```python
from build123d import *

# Parameters (mm, degrees)
F0_R     = 8.9
F3_DEPTH = 13.5
F0_W     = 27.7
F0_H     = 11
F0_H_2   = 1.2
F4_DEPTH = 10.5
F2_R     = 10.7
F5_DEPTH = 5
F2_R_2   = 3.25
F6_DEPTH = 2
F2_R_3   = 3
F7_DEPTH = 6
F8_DEPTH = 5.5
F9_SIZE  = 1
F10_SIZE = 2
F11_R    = 0.2


with BuildPart() as f3:
    # F0 (on Top) → F3 (new body)
    with BuildSketch(Plane.XY):
        with BuildLine():
            Line((0, 19.0066603875), (0, 0))
            Line((0, 0), (18.3, 0))
            Line((18.3, 0), (18.3, 18.5502631652))
            ThreePointArc((18.3, 18.5502631652), (17.5, 23.3), (18.3, 28.0497368348))
            Line((18.3, 28.0497368348), (18.3, 36.8))
            Line((18.3, 36.8), (0, 36.8))
            Line((0, 36.8), (0, 27.5933396125))
            Line((0, 27.5933396125), (3.4058666579, 26.680740392))
            ThreePointArc((3.4058666579, 26.680740392), (6, 23.3), (3.4058666579, 19.919259608))
            Line((3.4058666579, 19.919259608), (0, 19.0066603875))
        make_face()
        with BuildLine():
            Line((18.3, 18.5502631652), (18.3, 0))
            Line((18.3, 0), (35.3, 0))
            Line((35.3, 0), (35.3, 7))
            ThreePointArc((35.3, 7), (36.4715728753, 9.8284271247), (39.3, 11))
            Line((39.3, 11), (64.3, 11))
            Line((64.3, 11), (64.3, 35.6))
            Line((64.3, 35.6), (39.3, 35.6))
            ThreePointArc((39.3, 35.6), (37.7508066615, 35.9121822171), (36.4434286286, 36.8))
            Line((36.4434286286, 36.8), (18.3, 36.8))
            Line((18.3, 36.8), (18.3, 28.0497368348))
            ThreePointArc((18.3, 28.0497368348), (17.5, 23.3), (18.3, 18.5502631652))
        make_face()
        with Locations((32, 23.3)):
            Circle(F0_R, mode=Mode.SUBTRACT)
        with BuildLine():
            Line((64.3, 35.6), (64.3, 11))
            Line((64.3, 11), (92, 11))
            Line((92, 11), (92, 19.0066603875))
            Line((92, 19.0066603875), (88.5941333421, 19.919259608))
            ThreePointArc((88.5941333421, 19.919259608), (86, 23.3), (88.5941333421, 26.680740392))
            Line((88.5941333421, 26.680740392), (92, 27.5933396125))
            Line((92, 27.5933396125), (92, 35.6))
            Line((92, 35.6), (64.3, 35.6))
        make_face()
    extrude(amount=F3_DEPTH)

    # F0 (on Top) → F4 (join)
    with BuildSketch(Plane.XY):
        with BuildLine():
            Line((35.3, 7), (35.3, 0))
            Line((35.3, 0), (64.3, 0))
            Line((64.3, 0), (64.3, 11))
            Line((64.3, 11), (39.3, 11))
            ThreePointArc((39.3, 11), (36.4715728753, 9.8284271247), (35.3, 7))
        make_face()
        with Locations((78.15, 5.5)):
            Rectangle(F0_W, F0_H)
        with Locations((78.15, 36.2)):
            Rectangle(F0_W, F0_H_2)
        with BuildLine():
            Line((39.3, 35.6), (64.3, 35.6))
            Line((64.3, 35.6), (64.3, 36.8))
            Line((64.3, 36.8), (36.4434286286, 36.8))
            ThreePointArc((36.4434286286, 36.8), (37.7508066615, 35.9121822171), (39.3, 35.6))
        make_face()
    extrude(amount=F4_DEPTH)

    # F2 (on offset) → F5 (cut)
    with BuildSketch(Plane.XY.offset(13.5)):
        with Locations((32, 23.3)):
            Circle(F2_R)
    extrude(amount=-F5_DEPTH, mode=Mode.SUBTRACT)

    # F2 (on offset) → F6 (cut)
    with BuildSketch(Plane.XY.offset(13.5)):
        with Locations((50.6, 23.3)):
            Circle(F2_R_2)
    extrude(amount=-F6_DEPTH, mode=Mode.SUBTRACT)

    # F2 (on offset) → F7 (cut)
    with BuildSketch(Plane.XY.offset(13.5)):
        with Locations((32, 6.7)):
            Circle(F2_R_3)
    extrude(amount=-F7_DEPTH, mode=Mode.SUBTRACT)

    # F2 (on offset) → F8 (join)
    with BuildSketch(Plane.XY.offset(13.5)):
        with BuildLine():
            Line((0, 0), (18.3, 0))
            Line((18.3, 0), (18.3, 18.5502631652))
            ThreePointArc((18.3, 18.5502631652), (17.5, 23.3), (18.3, 28.0497368348))
            Line((18.3, 28.0497368348), (18.3, 36.8))
            Line((18.3, 36.8), (0, 36.8))
            Line((0, 36.8), (0, 27.5933396125))
            Line((0, 27.5933396125), (3.4058666579, 26.680740392))
            ThreePointArc((3.4058666579, 26.680740392), (6, 23.3), (3.4058666579, 19.919259608))
            Line((3.4058666579, 19.919259608), (0, 19.0066603875))
            Line((0, 19.0066603875), (0, 0))
        make_face()
        with BuildLine():
            Line((64.3, 35.6), (64.3, 11))
            Line((64.3, 11), (92, 11))
            Line((92, 11), (92, 19.0066603875))
            Line((92, 19.0066603875), (88.5941333421, 19.919259608))
            ThreePointArc((88.5941333421, 19.919259608), (86, 23.3), (88.5941333421, 26.680740392))
            Line((88.5941333421, 26.680740392), (92, 27.5933396125))
            Line((92, 27.5933396125), (92, 35.6))
            Line((92, 35.6), (64.3, 35.6))
        make_face()
    extrude(amount=F8_DEPTH)

    # F9
    f9_edges = [f3.edges().sort_by_distance(p)[0] for p in [
        (18.3, 9.275132, 19),
        (23.1, 23.3, 8.5),
        (64.3, 23.3, 19),
    ]]
    chamfer(f9_edges, length=F9_SIZE)

    # F10
    f10_edges = [f3.edges().sort_by_distance(p)[0] for p in [
        (92, 0, 5.25),
        (0, 0, 9.5),
        (92, 36.8, 5.25),
        (0, 36.8, 9.5),
    ]]
    chamfer(f10_edges, length=F10_SIZE)

    # F11
    f11_edges = [f3.edges().sort_by_distance(p)[0] for p in [
        (47.35, 23.3, 13.5),
        (35.3, 3.5, 13.5),
        (64.3, 11, 15.75),
        (64.8, 11, 18.5),
        (78.65, 11, 19),
        (92, 11, 14.75),
        (92, 6.5, 10.5),
        (91, 1, 10.5),
        (62.65, 0, 10.5),
        (35.3, 0, 12),
        (26.8, 0, 13.5),
        (18.3, 0, 15.75),
        (17.8, 0, 18.5),
        (9.65, 0, 19),
        (1, 1, 19),
        (0, 10.50333, 19),
        (1.702933, 19.46296, 19),
        (6, 23.3, 19),
        (0, 31.19667, 19),
        (1, 35.8, 19),
        (9.65, 36.8, 19),
        (17.8, 36.8, 18.5),
        (18.3, 36.8, 15.75),
        (27.371714, 36.8, 13.5),
        (92, 15.00333, 19),
        (90.297067, 19.46296, 19),
        (86, 23.3, 19),
        (90.297067, 27.13704, 19),
        (92, 31.19667, 19),
        (91.6, 35.2, 19),
        (78.25, 35.6, 19),
        (64.8, 35.6, 18.5),
        (64.3, 35.6, 15.75),
        (51.8, 35.6, 13.5),
        (37.750807, 35.912182, 13.5),
        (1, 1, 0),
        (46, 0, 0),
        (91, 1, 0),
        (92, 10.50333, 0),
        (90.297067, 19.46296, 0),
        (86, 23.3, 0),
        (92, 31.19667, 0),
        (91, 35.8, 0),
        (0, 10.50333, 0),
        (1.702933, 19.46296, 0),
        (6, 23.3, 0),
        (1.702933, 27.13704, 0),
        (0, 31.19667, 0),
        (1, 35.8, 0),
        (46, 36.8, 0),
    ]]
    fillet(f11_edges, radius=F11_R)


solid = f3.part
```
CAD build for the part. Positions are in the model's coordinates, mm. A direction names the side the tool comes from. Give positions to 0.01 mm unless a question says otherwise; leave off trailing zeros. Order: outer loops, then holes, each group sorted by start corner. A loop starts at its lowest first (then second) coordinate and runs counter-clockwise, first axis right, second up.
(1) Flat gauge pins, fed straight in: pin 1 (2 mm diameter, centred on x = 50.5, y = 21.5, fed in from -Z); pin 2 (10.5 mm diameter, centred on x = 32.5, y = 20, fed in from +Z); pin 3 (10 mm diameter, centred on x = 22.5, y = 32.5, fed in from +Z); pin 4 (5 mm diameter, centred on x = 33, y = 6.5, fed in from +Z). Where does each tip first touch, or does it go through?
(2) Tool access for faces 1 (the flat face through (71, 35.6, 14)), 2 (the cylindrical face through (23.5, 16.8, 11)), 3 (the flat face through (18.3, 9, 16)): list every direction of +Z, -Z, +X, -X, +Y, -Y with a clear straight run to the whole face (end or side of a thin tool).
(3) Drill centre lines: L1, parallel to Y at x = 32, z = 12; L2, parallel to Y at x = 32, z = 3.75; L3, parallel to Y at x = 50.6, z = 12.2. Where is each one in solid material? Low to high.
(4) Saw through at D-D, the plane x = 81.5. Give the cut face in (y, z).
(5) Saw through at C-C, the plane z = 3.5. Give the cut face in (x, y).
(6) Saw through at A-A, the plane x = 32. Give the cut face in (y, z), then the cut area to 3 significant figures.
(7) Mould opens along Y. For faces 4 (the flat face through (37, 36.8, 7)), 5 (the flat face through (92, 31, 9)), 6 (the flat face through (39, 16, 8.5)) say: released by +Y, released by -Y, zero draft, split by the parting line, or undercut.
Results found:
1. pin 1: stops at z = 0
1. pin 2: passes through
1. pin 3: stops at z = 18.8
1. pin 4: stops at z = 13.5
2. face 1: +Z, +X, +Y
2. face 2: +Z
2. face 3: +Z, +Y, -Y
3. L1: y = 0 to 3.7, 9.7 to 12.6, 34 to 36.8
3. L2: y = 0 to 14.4, 32.2 to 36.8
3. L3: y = 11 to 20.05, 26.55 to 35.6
4. outline: (0, 0.2) arc R0.2 ccw to (0.2, 0) - (36.6, 0) arc R0.2 ccw to (36.8, 0.2) - (36.8, 10.5) - (35.6, 10.5) - (35.6, 18.8) arc R0.2 ccw to (35.4, 19) - (11.2, 19) arc R0.2 ccw to (11, 18.8) - (11, 10.5) - (0.2, 10.5) arc R0.2 ccw to (0, 10.3) - close
5. outline: (0, 2) - (2, 0) - (90, 0) - (92, 2) - (92, 19.01) - (88.59, 19.92) arc R3.5 cw to (88.59, 26.68) - (92, 27.59) - (92, 34.8) - (90, 36.8) - (2, 36.8) - (0, 34.8) - (0, 27.59) - (3.41, 26.68) arc R3.5 cw to (3.41, 19.92) - (0, 19.01) - close; hole circle Ø17.8 at (32, 23.3)
6. outline: (0, 0.2) arc R0.2 ccw to (0.2, 0) - (14.4, 0) - (14.4, 7.5) - (13.4, 8.5) - (12.6, 8.5) - (12.6, 13.5) - (9.7, 13.5) - (9.7, 7.5) - (3.7, 7.5) - (3.7, 13.5) - (0.2, 13.5) arc R0.2 ccw to (0, 13.3) - close; (32.2, 0) - (36.6, 0) arc R0.2 ccw to (36.8, 0.2) - (36.8, 13.3) arc R0.2 ccw to (36.6, 13.5) - (34, 13.5) - (34, 8.5) - (33.2, 8.5) - (32.2, 7.5) - close
6. area: 201 mm2
7. face 4: released by +Y
7. face 5: zero draft
7. face 6: undercut
